```python
from build123d import *

# Parameters (mm, degrees)
F1_START = 6.4
F0_R     = 12.5
F1_DEPTH = 2.97
F2_R     = 8
F3_DEPTH = 6.4
F4_SIZE2 = 2.5
F4_SIZE  = 4
F5_R     = 4.25
F6_DEPTH = 9.37
F8_START = 2.35
F7_R     = 6.55
F8_DEPTH = 22.65


with BuildPart() as f1:
    # F0 (on Top) → F1 (new body)
    with BuildSketch(Plane.XY.offset(F1_START)):
        Circle(F0_R)
    extrude(amount=F1_DEPTH)

    # F2 (on Top) → F3 (join, through all)
    with BuildSketch(Plane.XY):
        Circle(F2_R)
    extrude(amount=F3_DEPTH)

    # F4
    f4_edges = [f1.edges().sort_by_distance(p)[0] for p in [
        (-12.5, 0, 9.37),
    ]]
    f4_side = f1.faces().sort_by_distance((0, 0, 9.37))[0]
    chamfer(f4_edges, length=F4_SIZE, length2=F4_SIZE2, reference=f4_side)

    # F5 (on Top) → F6 (cut, through all)
    with BuildSketch(Plane.XY):
        Circle(F5_R)
    extrude(amount=F6_DEPTH, mode=Mode.SUBTRACT)

    # F7 (on Top) → F8 (cut)
    with BuildSketch(Plane.XY.offset(F8_START)):
        Circle(F7_R)
    extrude(amount=F8_DEPTH, mode=Mode.SUBTRACT)


solid = f1.part
```
Geometry check sheet. Reference: the model listing, model coordinates, mm. A direction names the side the tool comes from. Give positions to 0.01 mm unless a question says otherwise; leave off trailing zeros. Order: outer loops, then holes, each group sorted by start corner. A loop starts at its lowest first (then second) coordinate and runs counter-clockwise, first axis right, second up. Notation, with made-up numbers: (-8, 25.5) - (25, 25.5) arc R29 ccw to (25, 50.5) - close; hole circle Ø6 at (46, -15.5). An arc over 180 degrees is marked (long way). Answer in a Markdown table with one row per item. Add a question column.
Q1. Mould release check, pull along X, two halves, no side actions. Record for faces 4 (the conical face through (8.35, 2.63, 9.21)), 5 (the flat face through (3.4, -3.4, 0)), 6 (the cylindrical face through (2.285, 3.584, 1.159)): pulls with the +X half, pulls with the -X half, needs draft (parallel to the pull), parting line crosses it, or undercut.
Q2. Gauge pin test, flat ends, axial feed: pin 1 (1 mm diameter, centred on x = 0.5, z = 7.5, fed in from +Y); pin 2 (1.5 mm diameter, centred on x = 7.5, z = 5.5, fed in from -Y); pin 3 (5 mm diameter, centred on y = -7, z = 6.5, fed in from -X). Record the tip position at first contact, or that the pin passes through.
Q3. Cross-section at A-A, the plane x = 0. Enter the section's corners in (y, z).
Q4. Material ranges on probe 1 along Y at (x, z) = (0, 0.5); probe 2 along X at (y, z) = (0.25, 1.5); probe 3 along Y at (x, z) = (0, 5.75), recorded low to high. Write a range as from..to.
Q5. Cross-section at D-D, the plane z = 1. Enter the section's corners in (x, y), then the cut area to 3 significant figures.
Q6. Tool access check on faces 1 (the cylindrical face through (-1.73, -7.81, 3.16)), 2 (the flat face through (2.5, -6.3, 9.37)), 3 (the flat face through (1.4, -4.3, 2.35)). Record the directions out of +Z, -Z, +X, -X, +Y, -Y that give a thin tool (end or side, any length) a straight path to the whole face; none if there is none.
Q7. Cross-section at C-C, the plane z = 5. Enter the section's corners in (x, y).
Check values:
| question | item | result |
|---|---|---|
| 1 | face 4 | parting line crosses it |
| 1 | face 5 | needs draft |
| 1 | face 6 | undercut |
| 2 | pin 1 | stops at y = 12.28 |
| 2 | pin 2 | stops at y = -4.29 |
| 2 | pin 3 | stops at x = -11.66 |
| 3 | outline | (-12.5, 6.4) - (-8, 6.4) - (-8, 0) - (-4.25, 0) - (-4.25, 2.35) - (-6.55, 2.35) - (-6.55, 9.37) - (-8.5, 9.37) - (-12.5, 6.87) - close; (4.25, 0) - (8, 0) - (8, 6.4) - (12.5, 6.4) - (12.5, 6.87) - (8.5, 9.37) - (6.55, 9.37) - (6.55, 2.35) - (4.25, 2.35) - close |
| 4 | probe 1 | y = -8..-4.25, 4.25..8 |
| 4 | probe 2 | x = -8..-4.24, 4.24..8 |
| 4 | probe 3 | y = -8..-6.55, 6.55..8 |
| 5 | outline | circle Ø16 at (0, 0); hole circle Ø8.5 at (0, 0) |
| 5 | area | 144 mm^2 |
| 6 | face 1 | -Z |
| 6 | face 2 | +Z, +X, -X, +Y, -Y |
| 6 | face 3 | +Z |
| 7 | outline | circle Ø16 at (0, 0); hole circle Ø13.1 at (0, 0) |
